CAD build for the part. Positions are in the model's coordinates, mm. Give positions to 0.01 mm unless a question says otherwise; leave off trailing zeros. Write each loop counter-clockwise with the first axis right and the second up, starting at its lowest first coordinate (ties: lowest second). Pieces come first, ordered by that corner, then holes. Notation, with made-up numbers: (80, -27) -> (131, -27) arc R22 ccw to (131, 6) -> close; hole circle Ø3 at (3.5, 56). An arc over 180 degrees is marked (long way). Answer in a Markdown table with one row per item. Add a question column.
```python
from build123d import *

# Parameters (mm, degrees)
SKETCH1_R           = 14.2875
SKETCH1_R_2         = 3.175
BOSS_EXTRUDE1_DEPTH = 6.35


with BuildPart() as part:
    # Sketch1 → Boss-Extrude1 (new body)
    with BuildSketch(Plane(origin=(0, 0, 0), x_dir=(0, 0, -1), z_dir=(1, 0, 0))):
        with BuildLine():
            Line((0, 25.4), (38.1, 25.4))
            Line((38.1, 25.4), (38.1, -25.4))
            Line((38.1, -25.4), (0, -25.4))
            ThreePointArc((0, -25.4), (-25.4, 0), (0, 25.4))
        make_face()
        Circle(SKETCH1_R, mode=Mode.SUBTRACT)
        with Locations((25.4, 15.875)):
            Circle(SKETCH1_R_2, mode=Mode.SUBTRACT)
        with Locations((25.4, -15.875)):
            Circle(SKETCH1_R_2, mode=Mode.SUBTRACT)
    extrude(amount=BOSS_EXTRUDE1_DEPTH)


solid = part.part
```
Item 1: Slice it at C-C, the plane z = 10.5. List the corners of the cut face in (x, y), then the cut area to 3 significant figures.
Item 2: Slice it at A-A, the plane y = 0. List the corners of the cut face in (x, z).
Item 3: Drop flat-ended pins along their axis: pin 1 Ø2 at (y, z) = (-18, -8) entering from -X; pin 2 Ø2 at (x, y) = (3, 4.5) entering from +Z; pin 3 Ø1.5 at (x, y) = (4.5, -19.5) entering from +Z. Give the stop position or say it passes through.
Item 4: Probe L1, parallel to Y at x = 3, z = -25.4; L2, parallel to Y at x = 2.5, z = -23.5; L3, parallel to Z at x = 5.5, y = -16. List the from-to ranges inside material, lowest first. Write a range as from..to.
Item 5: Slice it at B-B, the plane z = -25.4. List the corners of the cut face in (x, y), then the cut area to 3 significant figures.
Item 6: Mould opens along Y. For faces 1 (the face through (3.13, -14.92, -28.43)), 2 (the face through (3.131, -0.559, 25.394)), 3 (the face through (3, 25.4, -19)) say: released by +Y, released by -Y, zero draft, split by the parting line, or undercut.
Item 7: Slice it at D-D, the plane x = 1.25. State how many separate pieces and enclosed holes the cut face has, then the cut area to 3 significant figures.
Answer key:
| question | item | result |
|---|---|---|
| 1 | outline | (0, -23.13) -> (6.35, -23.13) -> (6.35, -9.69) -> (0, -9.69) -> close; (0, 9.69) -> (6.35, 9.69) -> (6.35, 23.13) -> (0, 23.13) -> close |
| 1 | area | 171 mm² |
| 2 | outline | (0, -38.1) -> (6.35, -38.1) -> (6.35, -14.29) -> (0, -14.29) -> close; (0, 14.29) -> (6.35, 14.29) -> (6.35, 25.4) -> (0, 25.4) -> close |
| 3 | pin 1 | stops at x = 0 |
| 3 | pin 2 | stops at z = 25.16 |
| 3 | pin 3 | stops at z = 17.13 |
| 4 | L1 | y = -25.4..-19.05, -12.7..12.7, 19.05..25.4 |
| 4 | L2 | y = -25.4..-18.42, -13.33..13.33, 18.42..25.4 |
| 4 | L3 | z = -38.1..-28.57, -22.23..19.73 |
| 5 | outline | (0, -25.4) -> (6.35, -25.4) -> (6.35, -19.05) -> (0, -19.05) -> close; (0, -12.7) -> (6.35, -12.7) -> (6.35, 12.7) -> (0, 12.7) -> close; (0, 19.05) -> (6.35, 19.05) -> (6.35, 25.4) -> (0, 25.4) -> close |
| 5 | area | 242 mm² |
| 6 | face 1 | undercut |
| 6 | face 2 | split by the parting line |
| 6 | face 3 | released by +Y |
| 7 | separate pieces | 1 |
| 7 | enclosed holes | 3 |
| 7 | area | 2,240 mm² |
